```python
from build123d import *

# Parameters (mm, degrees)
SKETCH1_R           = 3.225
BOSS_EXTRUDE1_DEPTH = 180


with BuildPart() as part:
    # Sketch1 → Boss-Extrude1 (new body)
    with BuildSketch(Plane(origin=(0, 0, 0), x_dir=(0, 0, -1), z_dir=(1, 0, 0))):
        with BuildLine():
            Line((-20.678840597, -3.225), (-7.321159403, -3.225))
            ThreePointArc((-7.321159403, -3.225), (0, 8), (7.321159403, -3.225))
            Line((7.321159403, -3.225), (7.321159403, -7.225))
            Line((7.321159403, -7.225), (-35.321159403, -7.225))
            Line((-35.321159403, -7.225), (-35.321159403, -3.225))
            ThreePointArc((-35.321159403, -3.225), (-28, 8), (-20.678840597, -3.225))
        make_face()
        Circle(SKETCH1_R, mode=Mode.SUBTRACT)
        with Locations((-28, 0)):
            Circle(SKETCH1_R, mode=Mode.SUBTRACT)
    extrude(amount=BOSS_EXTRUDE1_DEPTH)


solid = part.part
```
Could you check a few things on this model? Use its own coordinates, in mm. A direction names the side the tool comes from. Give positions to 0.01 mm unless a question says otherwise; leave off trailing zeros. Loops run counter-clockwise (first coordinate to the right, second up) from the corner with the lowest first, then second, coordinate; pieces in that order, holes last. Notation, with made-up numbers: (-24, -5.75) - (12, -5.75) arc R22 ccw to (12, 14.25) - close; hole circle Ø4 at (2, 52). An arc over 180 degrees is marked (long way). Answer in a Markdown table with one row per item. Add a question column.
Q1. Please list where these lines run through material, in increasing order: L1, parallel to Y at x = 143, z = 28 (3 decimals); L2, parallel to Z at x = 133, y = 0.5; L3, parallel to Z at x = 114.5, y = 2.75. Write a range as from..to.
Q2. If we section it at C-C (x = 104.5): List the corners of the cut face in (y, z) for me (3 decimals), plus the area to 3 significant figures.
Q3. Which directions (+Z, -Z, +X, -X, +Y, -Y) give clear straight access to the entire face, cutting with the end or side of a thin tool? Please do faces 4 (the face through (88.74, 0.14, 31.22)), 5 (the face through (89, -5, -7.321)).
Q4. We'd pull the mould along Y, two halves only. Please class faces 1 (the face through (89, -7.225, 14)), 2 (the face through (88.74, -3.15, 0.7)), 3 (the face through (89, -5, 35.321)): +Y half, -Y half, draft (parallel to the pull), parting line (faces both ways), or undercut.
Q5. If we section it at A-A (y = 0): List the corners of the cut face in (x, z) for me (3 decimals).
Q6. For pin 1 (4 mm diameter, centred on x = 56, z = 15.5, fed in from +Y) (3 decimals); pin 2 (1.5 mm diameter, centred on x = 90.5, z = 2, fed in from +Y); pin 3 (2 mm diameter, centred on x = 82.5, y = -6, fed in from +Z), each with a flat end and sliding along its axis, tell me the tip position at first contact or that it passes through.
Q7. If we section it at B-B (z = 0): List the corners of the cut face in (x, y) for me (3 decimals), plus the area to 3 significant figures.
Q8. If we section it at D-D (z = 13.5): List the corners of the cut face in (x, y) for me (3 decimals).
The answers:
| question | item | result |
|---|---|---|
| 1 | L1 | y = -7.225..-3.225, 3.225..8 |
| 1 | L2 | z = -7.98..-3.19, 3.19..7.98, 20.02..24.81, 31.19..35.98 |
| 1 | L3 | z = -7.51..-1.68, 1.68..7.51, 20.49..26.32, 29.68..35.51 |
| 2 | outline | (-7.225, -7.321) - (-3.225, -7.321) arc R8 ccw (long way) to (-3.225, 7.321) - (-3.225, 20.679) arc R8 ccw (long way) to (-3.225, 35.321) - (-7.225, 35.321) - close; hole circle Ø6.45 at (0, 0); hole circle Ø6.45 at (0, 28) |
| 2 | area | 407 mm^2 |
| 3 | face 4 | +X, -X |
| 3 | face 5 | -Z, +X, -X, -Y |
| 4 | face 1 | -Y half |
| 4 | face 2 | undercut |
| 4 | face 3 | draft |
| 5 | outline | (0, -8) - (180, -8) - (180, -3.225) - (0, -3.225) - close; (0, 3.225) - (180, 3.225) - (180, 8) - (0, 8) - close; (0, 20) - (180, 20) - (180, 24.775) - (0, 24.775) - close; (0, 31.225) - (180, 31.225) - (180, 36) - (0, 36) - close |
| 6 | pin 1 | stops at y = -3.225 |
| 6 | pin 2 | stops at y = 7.9 |
| 6 | pin 3 | stops at z = 35.32 |
| 7 | outline | (0, -7.225) - (180, -7.225) - (180, -3.225) - (0, -3.225) - close; (0, 3.225) - (180, 3.225) - (180, 8) - (0, 8) - close |
| 7 | area | 1,580 mm^2 |
| 8 | outline | (0, -7.225) - (180, -7.225) - (180, -3.225) - (0, -3.225) - close |
